Read the model definition and answer for the solid it produces. Units are mm, in the model's axes. Round coordinates to 2 decimals unless told otherwise and drop trailing zeros. Write each loop counter-clockwise with the first axis right and the second up, starting at its lowest first coordinate (ties: lowest second). Pieces come first, ordered by that corner, then holes. Notation, with made-up numbers: (25.5, -33) - (56.5, -33) arc R20 cw to (56.5, -22) - close; hole circle Ø10 at (85, -28.5). An arc over 180 degrees is marked (long way). Answer as CSV lines item,"result". Start each with the question number.
1) Find section A-A on x = 39.5. Determine the outline of the cut face in (y, z) (3 decimals), then the cut area to 3 significant figures.
2) Consider line 1 along X through (y, z) = (-2.5, -24); line 2 along Z through (x, y) = (-58.5, -1.5); line 3 along Z through (x, y) = (-23.5, -0.7). Determine where each line is inside the solid, lowest interval first.
3) Find section B-B on z = -33. Determine the outline of the cut face in (x, y) (3 decimals).
4) Find section C-C on y = -0.6. State how many separate pieces and enclosed holes the cut face has, then the cut area to 3 significant figures.
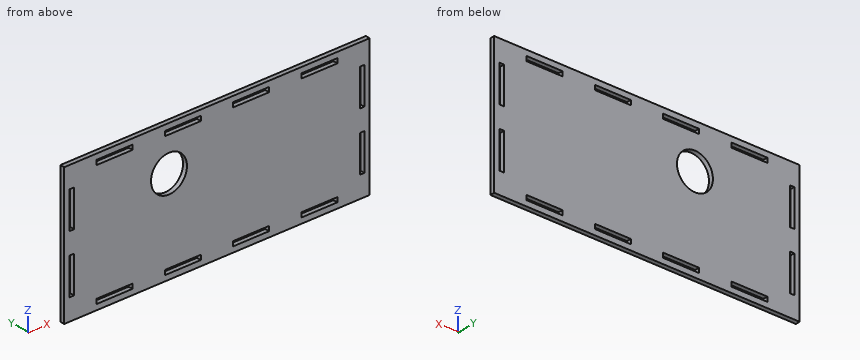
from build123d import *

# Parameters (mm, degrees)
F0_W     = 215.9
F0_H     = 95.25
F0_W_2   = 25.4254
F0_H_2   = 3.2004
F0_W_3   = 3.2004
F0_H_3   = 25.4254
F0_R     = 12.7
F1_DEPTH = 3.175


with BuildPart() as f1:
    # F0 (on Front) → F1 (new body)
    with BuildSketch(Plane.XZ):
        with Locations((10.806967, -3.292766)):
            Rectangle(F0_W, F0_H)
        with Locations((-61.590653, -45.507566)):
            Rectangle(F0_W_2, F0_H_2, mode=Mode.SUBTRACT)
        with Locations((-13.325573, -45.507566)):
            Rectangle(F0_W_2, F0_H_2, mode=Mode.SUBTRACT)
        with Locations((-91.732833, -23.407026)):
            Rectangle(F0_W_3, F0_H_3, mode=Mode.SUBTRACT)
        with Locations((34.939507, -45.507566)):
            Rectangle(F0_W_2, F0_H_2, mode=Mode.SUBTRACT)
        with Locations((83.204587, -45.507566)):
            Rectangle(F0_W_2, F0_H_2, mode=Mode.SUBTRACT)
        with Locations((113.346767, -23.407026)):
            Rectangle(F0_W_3, F0_H_3, mode=Mode.SUBTRACT)
        with Locations((-91.732833, 16.818954)):
            Rectangle(F0_W_3, F0_H_3, mode=Mode.SUBTRACT)
        with Locations((-23.097243, 13.552523)):
            Circle(F0_R, mode=Mode.SUBTRACT)
        with Locations((-61.590653, 38.922034)):
            Rectangle(F0_W_2, F0_H_2, mode=Mode.SUBTRACT)
        with Locations((-13.325573, 38.922034)):
            Rectangle(F0_W_2, F0_H_2, mode=Mode.SUBTRACT)
        with Locations((113.346767, 16.818954)):
            Rectangle(F0_W_3, F0_H_3, mode=Mode.SUBTRACT)
        with Locations((34.939507, 38.922034)):
            Rectangle(F0_W_2, F0_H_2, mode=Mode.SUBTRACT)
        with Locations((83.204587, 38.922034)):
            Rectangle(F0_W_2, F0_H_2, mode=Mode.SUBTRACT)
    extrude(amount=F1_DEPTH)


solid = f1.part
Check values:
1,outline,"(-3.175, -50.918) - (0, -50.918) - (0, -47.108) - (-3.175, -47.108) - close; (-3.175, -43.907) - (0, -43.907) - (0, 37.322) - (-3.175, 37.322) - close; (-3.175, 40.522) - (0, 40.522) - (0, 44.332) - (-3.175, 44.332) - close"
1,area,"282 mm^2"
2,line 1,"x = -97.14 to -93.33, -90.13 to 111.75, 114.95 to 118.76"
2,line 2,"z = -50.92 to -47.11, -43.91 to 37.32, 40.52 to 44.33"
2,line 3,"z = -50.92 to -47.11, -43.91 to 0.86, 26.25 to 37.32, 40.52 to 44.33"
3,outline,"(-97.143, -3.175) - (-93.333, -3.175) - (-93.333, 0) - (-97.143, 0) - close; (-90.133, -3.175) - (111.747, -3.175) - (111.747, 0) - (-90.133, 0) - close; (114.947, -3.175) - (118.757, -3.175) - (118.757, 0) - (114.947, 0) - close"
4,separate pieces,"1"
4,enclosed holes,"13"
4,area,"19,100 mm^2"
